from build123d import *

# Parameters (mm, degrees)
SKETCH2_R           = 17.4625
BOSS_EXTRUDE1_DEPTH = 18
SKETCH13_R          = 0.8
CUT_EXTRUDE6_DEPTH  = 7.3
SKETCH16_R          = 11
CUT_EXTRUDE9_DEPTH  = 15
CUT_EXTRUDE11_DEPTH = 22
SKETCH21_W          = 16.25
SKETCH21_H          = 2.78436417
CUT_EXTRUDE12_DEPTH = 31.559414466
CUT_EXTRUDE13_REACH = 32.559
SKETCH24_W          = 16.25
SKETCH24_H          = 6.70136321
CUT_EXTRUDE14_DEPTH = 17
SKETCH27_W          = 18.82071266
SKETCH27_H          = 0.75
CUT_EXTRUDE15_DEPTH = 31.559414466


with BuildPart() as part:
    # Sketch2 → Boss-Extrude1 (new body)
    with BuildSketch(Plane.XY):
        Circle(SKETCH2_R)
    extrude(amount=BOSS_EXTRUDE1_DEPTH)

    # Sketch13 → Cut-Extrude6 (cut)
    with BuildSketch(Plane.XY.offset(18)):
        with Locations((0, 13.5)):
            Circle(SKETCH13_R)
        with Locations((11.691342951, -6.75)):
            Circle(SKETCH13_R)
        with Locations((-11.691342951, -6.75)):
            Circle(SKETCH13_R)
    extrude(amount=-CUT_EXTRUDE6_DEPTH, mode=Mode.SUBTRACT)

    # Sketch16 → Cut-Extrude9 (cut)
    with BuildSketch(Plane.XY.offset(18)):
        Circle(SKETCH16_R)
    extrude(amount=-CUT_EXTRUDE9_DEPTH, mode=Mode.SUBTRACT)

    # Sketch20 → Cut-Extrude11 (cut)
    with BuildSketch(Plane(origin=(5.95728493, 0, -11.08430825), x_dir=(0, 0, 1), z_dir=(0, 1, 0))):
        Polygon((16.52930825, -11.021800725), (16.52930825, -6.906800725), (14.92930825, -6.906800725), (14.92930825, -4.926800725), (16.52930825, -4.926800725), (16.52930825, -0.811800725), (18.05430825, -0.811800725), (18.05430825, 1.028199275), (22.11430825, 1.028199275), (22.11430825, -0.811800725), (23.63930825, -0.811800725), (23.63930825, -11.021800725), (22.11430825, -11.021800725), (22.11430825, -12.861800725), (18.05430825, -12.861800725), (18.05430825, -11.021800725), align=None)
    extrude(amount=-CUT_EXTRUDE11_DEPTH, mode=Mode.SUBTRACT)

    # Sketch21 → Cut-Extrude12 (cut, through all)
    with BuildSketch(Plane.XY.offset(18)):
        with Locations((0, -16.852182085)):
            Rectangle(SKETCH21_W, SKETCH21_H)
    extrude(amount=-CUT_EXTRUDE12_DEPTH, mode=Mode.SUBTRACT)

    # Cut-Extrude13: up to this face of the body (flat: up to its plane)
    cut_extrude13_end = Plane(part.part.faces().sort_by_distance((0, 0, 3))[0])
    # Sketch24 → Cut-Extrude13 (cut, up to the picked face)
    with BuildSketch(Plane.XY.offset(18), mode=Mode.PRIVATE) as cut_extrude13_sk1:
        with Locations((0.005436819, -10.109318395)):
            Rectangle(SKETCH24_W, SKETCH24_H)
    cut_extrude13_tool1 = split(extrude(cut_extrude13_sk1.sketch, amount=-CUT_EXTRUDE13_REACH, mode=Mode.PRIVATE), bisect_by=cut_extrude13_end, keep=Keep.BOTH, mode=Mode.PRIVATE)
    add(cut_extrude13_tool1.solids().sort_by(Axis((0.005437, -10.109318, 18), (0, 0, -1)))[0], mode=Mode.SUBTRACT)

    # Sketch26 → Cut-Extrude14 (cut)
    with BuildSketch(Plane.XY.offset(18)):
        Polygon((-8.119563181, -13.71), (-8.119563181, -15.46), (8.119563181, -15.46), (8.119563181, -13.71), (8.930436819, -13.71), (8.930436819, -12.71), (-8.919563181, -12.71), (-8.919563181, -13.71), align=None)
    extrude(amount=-CUT_EXTRUDE14_DEPTH, mode=Mode.SUBTRACT)

    # Sketch27 → Cut-Extrude15 (cut, through all)
    with BuildSketch(Plane.XY.offset(18)):
        with Locations((0, -15.085)):
            Rectangle(SKETCH27_W, SKETCH27_H)
    extrude(amount=-CUT_EXTRUDE15_DEPTH, mode=Mode.SUBTRACT)


solid = part.part
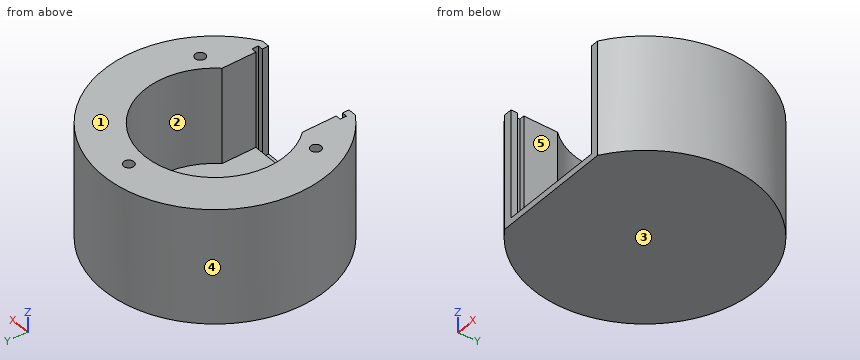
Geometry: final body of the model. Coordinates: model frame, mm. Face numbers are marked on the shaded views. A direction names the side the tool comes from. Coordinates: 2 decimals unless noted, no trailing zeros. Order: outer loops, then holes, each group sorted by start corner. A loop starts at its lowest first (then second) coordinate and runs counter-clockwise, first axis right, second up.
(1) Material intervals for probe 1 along X at (y, z) = (0, 14); probe 2 along Y at (x, z) = (8.5, 1.5); probe 3 along Z at (x, y) = (1.5, 10), sorted ascending.
(2) Section query A-A (z = 16). State how many separate pieces and enclosed holes the cut face has, plus the area to 3 significant figures.
(3) Section query C-C (x = 0). Return the cut outline in (y, z).
(4) Access query for the marked faces 1 and 2. Directions: +Z, -Z, +X, -X, +Y, -Y. A direction counts if a zero-diameter tool reaches every point of the face in a straight line with its end or side. Return the directions, or none.
(5) Section query D-D (z = 6.5). Return the cut outline in (x, y) (1 decimal).
(6) Section query B-B (y = 0). Return the cut outline in (x, z).
(7) First-contact query: pin 1 (5 mm diameter, centred on x = 3.5, z = 9, fed in from -Y); pin 2 (0.8 mm diameter, centred on x = 0, y = 13.5, fed in from +Z); pin 3 (6 mm diameter, centred on y = -10, z = 7.5, fed in from -X). Flat tips, straight axial feed; report the tip coordinate or a pass-through.
(8) Draft query along X for the marked faces 3, 4 and 5. Return one class per face: pulls with the +X half, pulls with the -X half, needs draft (parallel to the pull), parting line crosses it, or undercut.
Solution:
1. probe 1: x = -17.46 to -11, 11 to 17.46
1. probe 2: y = -14.71 to -13.71, -12.71 to 15.25
1. probe 3: z = 0 to 3
2. separate pieces: 1
2. enclosed holes: 3
2. area: 457 mm2
3. outline: (-14.71, 0) - (17.46, 0) - (17.46, 18) - (14.3, 18) - (14.3, 10.7) - (12.7, 10.7) - (12.7, 18) - (11, 18) - (11, 3) - (-12.71, 3) - (-12.71, 1) - (-14.71, 1) - close
4. face 1: +Z, +X, -X, +Y, -Y
4. face 2: +Z
5. outline: (-9.4, -14.7) - (-8.1, -14.7) - (-8.1, -13.7) - (-8.9, -13.7) - (-8.9, -12.7) - (-8.1, -12.7) - (-8.1, -7.4) arc R11 cw (long way) to (8.1, -7.4) - (8.1, -12.7) - (8.9, -12.7) - (8.9, -13.7) - (8.1, -13.7) - (8.1, -14.7) - (9.4, -14.7) arc R17.5 ccw (long way) to start
6. outline: (-17.46, 0) - (17.46, 0) - (17.46, 18) - (11, 18) - (11, 3) - (-11, 3) - (-11, 18) - (-17.46, 18) - close
7. pin 1: stops at y = 9.22
7. pin 2: stops at z = 10.7
7. pin 3: stops at x = -16
8. face 3: needs draft
8. face 4: parting line crosses it
8. face 5: undercut
